Verification items for the finished model (mm, model axes). Face numbers are marked on the shaded views. A direction names the side the tool comes from. Round coordinates to 2 decimals unless told otherwise and drop trailing zeros. Write each loop counter-clockwise with the first axis right and the second up, starting at its lowest first coordinate (ties: lowest second). Pieces come first, ordered by that corner, then holes. Notation, with made-up numbers: M 57.25,64 L 93.25,64 A17 ccw 93.25,69 Z; hole C 78.25,-16.75 d4. An arc over 180 degrees is marked long. Use a Markdown table: item, result. Add a question column.
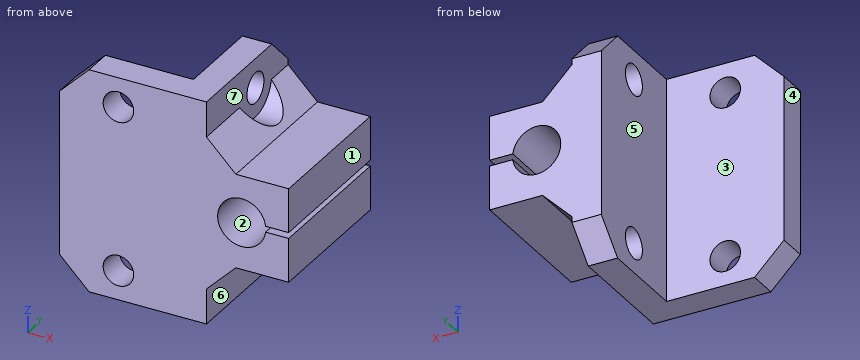
from build123d import *

# Parameters (mm, degrees)
SKETCH1_W           = 20
SKETCH1_H           = 38
SKETCH1_R           = 2.6
BOSS_EXTRUDE1_DEPTH = 5
SKETCH1_4_W         = 5
SKETCH1_4_H         = 38
BOSS_EXTRUDE2_DEPTH = 25
CHAMFER1_SIZE       = 5
SKETCH2_R           = 2.6
CUT_EXTRUDE1_DEPTH  = 20
SKETCH3_R           = 5
CUT_EXTRUDE2_DEPTH  = 15
CHAMFER2_SIZE       = 5
CHAMFER3_SIZE       = 5


with BuildPart() as part:
    # Sketch1 → Boss-Extrude1 (new body)
    with BuildSketch(Plane(origin=(0, 0, 0), x_dir=(1, 0, 0), z_dir=(0, 1, 0))):
        with Locations((10, -19)):
            Rectangle(SKETCH1_W, SKETCH1_H)
        with Locations((10, -33)):
            Circle(SKETCH1_R, mode=Mode.SUBTRACT)
        with Locations((10, -5)):
            Circle(SKETCH1_R, mode=Mode.SUBTRACT)
    extrude(amount=BOSS_EXTRUDE1_DEPTH)

    # Sketch1_4 → Boss-Extrude2 (add)
    with BuildSketch(Plane(origin=(0, 0, 0), x_dir=(1, 0, 0), z_dir=(0, 1, 0))):
        with Locations((22.5, -19)):
            Rectangle(SKETCH1_4_W, SKETCH1_4_H)
        with BuildLine():
            Line((39, -11), (25, -11))
            Line((25, -11), (25, -27))
            Line((25, -27), (39, -27))
            Line((39, -27), (39, -19.5))
            Line((39, -19.5), (35.06939799, -19.5))
            ThreePointArc((35.06939799, -19.5), (26.9, -19), (35.06939799, -18.5))
            Line((35.06939799, -18.5), (39, -18.5))
            Line((39, -18.5), (39, -11))
        make_face()
    extrude(amount=BOSS_EXTRUDE2_DEPTH)

    # Chamfer1
    chamfer1_edges = [part.edges().sort_by_distance(p)[0] for p in [
        (25, 12.5, 11),
        (25, 12.5, 27),
    ]]
    chamfer(chamfer1_edges, length=CHAMFER1_SIZE)

    # Sketch2 → Cut-Extrude1 (cut, through all)
    with BuildSketch(Plane.ZY.offset(-20)):
        with Locations((5, 15)):
            Circle(SKETCH2_R)
        with Locations((33, 15)):
            Circle(SKETCH2_R)
    extrude(amount=-CUT_EXTRUDE1_DEPTH, mode=Mode.SUBTRACT)

    # Sketch3 → Cut-Extrude2 (cut, through all)
    with BuildSketch(Plane.ZY.offset(-25)):
        with Locations((5, 15)):
            Circle(SKETCH3_R)
        with Locations((33, 15)):
            Circle(SKETCH3_R)
    extrude(amount=-CUT_EXTRUDE2_DEPTH, mode=Mode.SUBTRACT)

    # Chamfer2
    chamfer2_edges = [part.edges().sort_by_distance(p)[0] for p in [
        (22.5, 25, 0),
        (22.5, 25, 38),
    ]]
    chamfer(chamfer2_edges, length=CHAMFER2_SIZE)

    # Chamfer3
    chamfer3_edges = [part.edges().sort_by_distance(p)[0] for p in [
        (0, 2.5, 38),
        (0, 2.5, 0),
    ]]
    chamfer(chamfer3_edges, length=CHAMFER3_SIZE)


solid = part.part
1. Cross-section at A-A on x = 10. Enter the section's corners in (y, z), plus the area to 3 significant figures.
2. Cross-section at B-B on x = 31. Enter the section's corners in (y, z), plus the area to 3 significant figures.
3. Depth check by flat-ended pin: pin 1 Ø7 at (x, y) = (33, 15) entering from -Z; pin 2 Ø4 at (x, z) = (10, 33) entering from +Y; pin 3 Ø6 at (y, z) = (15, 5) entering from +X; pin 4 Ø4.5 at (x, y) = (37, 7) entering from +Z. Enter the tip coordinate at first touch or a pass-through.
4. Access from +Z, -Z, +X, -X, +Y, -Y to the whole of each face (thin tool, end or side, straight path). Record for the marked faces 5, 6 and 7.
5. Cross-section at C-C on y = 15. Enter the section's corners in (x, z).
6. Cross-section at D-D on x = 22.5. Enter the section's corners in (y, z), plus the area to 3 significant figures.
7. Scan lines: line 1 along Y through (x, z) = (21, 33); line 2 along Z through (x, y) = (10, 1.05); line 3 along X through (y, z) = (2.5, 5). Record each from-to range of solid material in increasing order. Write a range as from..to.
8. Release check for a two-part mould opening along X. For the marked faces 1, 2, 3 and 4 record: +X half, -X half, draft (parallel to the pull), parting line (faces both ways), or undercut.
Answer:
| question | item | result |
|---|---|---|
| 1 | outline | M 0,0 L 5,0 L 5,2.4 L 0,2.4 Z; M 0,7.6 L 5,7.6 L 5,30.4 L 0,30.4 Z; M 0,35.6 L 5,35.6 L 5,38 L 0,38 Z |
| 1 | area | 138 mm^2 |
| 2 | outline | M 0,11 L 25,11 L 25,14.9 L 0,14.9 Z; M 0,23.1 L 25,23.1 L 25,27 L 0,27 Z |
| 2 | area | 195 mm^2 |
| 3 | pin 1 | stops at z = 10.5 |
| 3 | pin 2 | passes through |
| 3 | pin 3 | stops at x = 25 |
| 3 | pin 4 | stops at z = 27 |
| 4 | face 5 | +Z, -Z, -X, +Y |
| 4 | face 6 | -Z, +X |
| 4 | face 7 | +Z, +X |
| 5 | outline | M 20,0 L 25,0 L 25,2.4 L 20,2.4 Z; M 20,7.6 L 25,7.6 L 25,10 L 29,10 L 30,11 L 39,11 L 39,18.5 L 35.07,18.5 A4.1 cw long 35.07,19.5 L 39,19.5 L 39,27 L 30,27 L 29,28 L 25,28 L 25,30.4 L 20,30.4 Z; M 20,35.6 L 25,35.6 L 25,38 L 20,38 Z |
| 6 | outline | M 0,0 L 20,0 L 25,5 L 25,33 L 20,38 L 0,38 Z; hole C 15,5 d5.2; hole C 15,33 d5.2 |
| 6 | area | 883 mm^2 |
| 7 | line 1 | y = 0..12.4, 17.6..25 |
| 7 | line 2 | z = 0..2.4, 7.6..30.4, 35.6..38 |
| 7 | line 3 | x = 0..7.4, 12.6..25 |
| 8 | face 1 | +X half |
| 8 | face 2 | undercut |
| 8 | face 3 | draft |
| 8 | face 4 | -X half |
